from build123d import *

# Parameters (mm, degrees)
EXTRUDE_1_DEPTH      = 5
SKETCH_2_R           = 3.25
CUT_EXTRUDE_1_DEPTH  = 5
SKETCH_10_R          = 1.75
CUT_EXTRUDE_8_DEPTH  = 45
SKETCH_11_R          = 3.5
CUT_EXTRUDE_9_DEPTH  = 3
SKETCH_12_W          = 44
SKETCH_12_H          = 44
CUT_EXTRUDE_10_DEPTH = 5
SKETCH_13_W          = 44
SKETCH_13_H          = 44
EXTRUDE_2_DEPTH      = 16
EXTRUDE_3_DEPTH      = 4
FILLET_1_R           = 5
SKETCH_16_R          = 11.5
CUT_EXTRUDE_11_DEPTH = 3
SKETCH_17_R          = 3
CUT_EXTRUDE_12_DEPTH = 3
FILLET_2_R           = 5
SKETCH_20_R          = 3
CUT_EXTRUDE_14_DEPTH = 39
EXTRUDE_START        = 20
SKETCH_21_R          = 4.5
SKETCH_21_R_2        = 3
EXTRUDE_4_DEPTH      = 20
CHAMFER_1_SIZE       = 10
CHAMFER_1_SIZE2      = 17.320508076
SKETCH_22_R          = 10
CUT_EXTRUDE_15_DEPTH = 2
SKETCH_23_R          = 4.5
CUT_EXTRUDE_16_DEPTH = 5


with BuildPart() as part:
    # 草图1 → 凸台-拉伸1 (new body)
    with BuildSketch(Plane(origin=(0, 0, 0), x_dir=(1, 0, 0), z_dir=(0, 1, 0))):
        with BuildLine():
            Line((-40, 104.403065089), (-40, 230))
            ThreePointArc((-40, 230), (0, 270), (40, 230))
            Line((40, 230), (40, 104.403065089))
            ThreePointArc((40, 104.403065089), (42.277916175, 56.729935627), (49.090909091, 9.491187735))
            ThreePointArc((49.090909091, 9.491187735), (0, -50), (-49.090909091, 9.491187735))
            ThreePointArc((-49.090909091, 9.491187735), (-42.277916175, 56.729935627), (-40, 104.403065089))
        make_face()
    extrude(amount=EXTRUDE_1_DEPTH)

    # 草图2 → 切除-拉伸1 (cut)
    with BuildSketch(Plane(origin=(0, 5, 0), x_dir=(1, 0, 0), z_dir=(0, 1, 0))):
        with Locations(Location((28.284271247, 28.284271247, 0), (0, 0, 270))):
            Circle(SKETCH_2_R)
        with Locations(Location((28.284271247, -28.284271247, 0), (0, 0, 270))):
            Circle(SKETCH_2_R)
        with Locations(Location((-28.284271247, -28.284271247, 0), (0, 0, 270))):
            Circle(SKETCH_2_R)
        with Locations(Location((-28.284271247, 28.284271247, 0), (0, 0, 270))):
            Circle(SKETCH_2_R)
    extrude(amount=-CUT_EXTRUDE_1_DEPTH, mode=Mode.SUBTRACT)

    # 草图10 → 切除-拉伸8 (cut)
    with BuildSketch(Plane.XZ):
        with Locations(Location((46, 0, 0), (0, 0, 270))):
            Circle(SKETCH_10_R)
        with Locations(Location((36, -104.403065089, 0), (0, 0, 270))):
            Circle(SKETCH_10_R)
        with Locations(Location((36, -230, 0), (0, 0, 270))):
            Circle(SKETCH_10_R)
        with Locations(Location((-36, -230, 0), (0, 0, 270))):
            Circle(SKETCH_10_R)
        with Locations(Location((-36, -104.403065089, 0), (0, 0, 270))):
            Circle(SKETCH_10_R)
        with Locations(Location((-46, 0, 0), (0, 0, 270))):
            Circle(SKETCH_10_R)
    extrude(amount=-CUT_EXTRUDE_8_DEPTH, mode=Mode.SUBTRACT)

    # 草图11 → 切除-拉伸9 (cut)
    with BuildSketch(Plane(origin=(0, 5, 0), x_dir=(1, 0, 0), z_dir=(0, 1, 0))):
        with Locations(Location((-36, 230, 0), (0, 0, 270))):
            Circle(SKETCH_11_R)
        with Locations(Location((-36, 104.403065089, 0), (0, 0, 270))):
            Circle(SKETCH_11_R)
        with Locations(Location((-46, 0, 0), (0, 0, 270))):
            Circle(SKETCH_11_R)
        with Locations(Location((46, 0, 0), (0, 0, 90))):
            Circle(SKETCH_11_R)
        with Locations(Location((36, 104.403065089, 0), (0, 0, 90))):
            Circle(SKETCH_11_R)
        with Locations(Location((36, 230, 0), (0, 0, 90))):
            Circle(SKETCH_11_R)
    extrude(amount=-CUT_EXTRUDE_9_DEPTH, mode=Mode.SUBTRACT)

    # 草图12 → 切除-拉伸10 (cut)
    with BuildSketch(Plane(origin=(0, 5, 0), x_dir=(1, 0, 0), z_dir=(0, 1, 0))):
        with Locations((0, -4)):
            Rectangle(SKETCH_12_W, SKETCH_12_H)
    extrude(amount=-CUT_EXTRUDE_10_DEPTH, mode=Mode.SUBTRACT)

    # 草图13 → 凸台-拉伸2 (add)
    with BuildSketch(Plane.XZ):
        with BuildLine():
            Line((-21, 30), (21, 30))
            ThreePointArc((21, 30), (24.535533906, 28.535533906), (26, 25))
            Line((26, 25), (26, -17))
            ThreePointArc((26, -17), (24.535533906, -20.535533906), (21, -22))
            Line((21, -22), (-21, -22))
            ThreePointArc((-21, -22), (-24.535533906, -20.535533906), (-26, -17))
            Line((-26, -17), (-26, 25))
            ThreePointArc((-26, 25), (-24.535533906, 28.535533906), (-21, 30))
        make_face()
        with Locations((0, 4)):
            Rectangle(SKETCH_13_W, SKETCH_13_H, mode=Mode.SUBTRACT)
    extrude(amount=EXTRUDE_2_DEPTH)

    # 草图15 → 凸台-拉伸3 (add)
    with BuildSketch(Plane.XZ.offset(16)):
        with BuildLine():
            Line((26, -17), (26, 25))
            ThreePointArc((26, 25), (24.535533906, 28.535533906), (21, 30))
            Line((21, 30), (-21, 30))
            ThreePointArc((-21, 30), (-24.535533906, 28.535533906), (-26, 25))
            Line((-26, 25), (-26, -17))
            ThreePointArc((-26, -17), (-24.535533906, -20.535533906), (-21, -22))
            Line((-21, -22), (21, -22))
            ThreePointArc((21, -22), (24.535533906, -20.535533906), (26, -17))
        make_face()
    extrude(amount=EXTRUDE_3_DEPTH)

    # 圆角1
    fillet_1_edges = [part.edges().sort_by_distance(p)[0] for p in [
        (24.535533906, -20, 28.535533906),
        (0, -20, 30),
        (-24.535533906, -20, 28.535533906),
        (-26, -20, 4),
        (-24.535533906, -20, -20.535533906),
        (0, -20, -22),
        (24.535533906, -20, -20.535533906),
        (26, -20, 4),
    ]]
    fillet(fillet_1_edges, radius=FILLET_1_R)

    # 草图16 → 切除-拉伸11 (cut)
    with BuildSketch(Plane(origin=(0, -16, 0), x_dir=(1, 0, 0), z_dir=(0, 1, 0))):
        with Locations(Location((0, -4, 0), (0, 0, 270))):
            Circle(SKETCH_16_R)
    extrude(amount=-CUT_EXTRUDE_11_DEPTH, mode=Mode.SUBTRACT)

    # 草图17 → 切除-拉伸12 (cut)
    with BuildSketch(Plane(origin=(0, -19, 0), x_dir=(1, 0, 0), z_dir=(0, 1, 0))):
        with Locations(Location((0, -4, 0), (0, 0, 270))):
            Circle(SKETCH_17_R)
    extrude(amount=-CUT_EXTRUDE_12_DEPTH, mode=Mode.SUBTRACT)

    # 圆角2
    fillet_2_edges = [part.edges().sort_by_distance(p)[0] for p in [
        (22, -5.5, -18),
        (22, -5.5, 26),
        (-22, -5.5, 26),
        (-22, -5.5, -18),
    ]]
    fillet(fillet_2_edges, radius=FILLET_2_R)

    # 草图20 → 切除-拉伸14 (cut)
    with BuildSketch(Plane.XZ):
        with Locations(Location((0, -230, 0), (0, 0, 270))):
            Circle(SKETCH_20_R)
    extrude(amount=-CUT_EXTRUDE_14_DEPTH, mode=Mode.SUBTRACT)

    # 草图21 → 凸台-拉伸4 (add)
    with BuildSketch(Plane.XZ.offset(EXTRUDE_START)):
        with Locations(Location((0, -230, 0), (0, 0, 270))):
            Circle(SKETCH_21_R)
        with Locations(Location((0, -230, 0), (0, 0, 270))):
            Circle(SKETCH_21_R_2, mode=Mode.SUBTRACT)
    extrude(amount=-EXTRUDE_4_DEPTH)

    # 倒角1
    chamfer_1_edges = [part.edges().sort_by_distance(p)[0] for p in [
        (0, 0, -225.5),
    ]]
    chamfer_1_side = [part.faces().sort_by_distance(p)[0] for p in [
        (0, 0, -117.507600063),
    ]]
    chamfer(chamfer_1_edges, length=CHAMFER_1_SIZE, length2=CHAMFER_1_SIZE2, reference=chamfer_1_side[0])

    # 草图22 → 切除-拉伸15 (cut)
    with BuildSketch(Plane(origin=(0, 5, 0), x_dir=(1, 0, 0), z_dir=(0, 1, 0))):
        with Locations(Location((0, 230, 0), (0, 0, 270))):
            Circle(SKETCH_22_R)
    extrude(amount=-CUT_EXTRUDE_15_DEPTH, mode=Mode.SUBTRACT)

    # 草图23 → 切除-拉伸16 (cut)
    with BuildSketch(Plane(origin=(0, 5, 0), x_dir=(1, 0, 0), z_dir=(0, 1, 0))):
        with Locations(Location((0, 28.284271247, 0), (0, 0, 270))):
            Circle(SKETCH_23_R)
    extrude(amount=-CUT_EXTRUDE_16_DEPTH, mode=Mode.SUBTRACT)


solid = part.part
CAD build for the part. Positions are in the model's coordinates, mm. A direction names the side the tool comes from. Coordinates: 2 decimals unless noted, no trailing zeros. Order: outer loops, then holes, each group sorted by start corner. A loop starts at its lowest first (then second) coordinate and runs counter-clockwise, first axis right, second up. Notation, with made-up numbers: (11.5, -39.75) -> (29.5, -39.75) arc R17 cw to (29.5, -34.75) -> close; hole circle Ø4 at (66, 22). An arc over 180 degrees is marked (long way). Answer in a Markdown table with one row per item.
1) Band-saw the part on B-B (z = -208). List the corners of the cut face in (x, y).
Check values:
| item | result |
|---|---|
| outline | (-40, 0) -> (40, 0) -> (40, 5) -> (-40, 5) -> close |
2) Flat gauge pins, fed straight in: P1, Ø1.5, axis at x = -29, z = -196, coming from the -Y side; P2, Ø2, axis at x = -44.5, z = -0.5, coming from the +Y side; P3, Ø10.5, axis at y = -5, z = 9, coming from the -X side. Where does each tip first touch, or does it go through?
Check values:
| item | result |
|---|---|
| P1 | y = 0 |
| P2 | y = 2 |
| P3 | x = -49.45 |
3) Band-saw the part on A-A (y = -11.5). List the corners of the cut face in (x, z).
Check values:
| item | result |
|---|---|
| outline | (-26, -17) arc R5 ccw to (-21, -22) -> (21, -22) arc R5 ccw to (26, -17) -> (26, 25) arc R5 ccw to (21, 30) -> (-21, 30) arc R5 ccw to (-26, 25) -> close; circle Ø15.72 at (0, -230); hole (-22, -13) arc R5 ccw to (-17, -18) -> (17, -18) arc R5 ccw to (22, -13) -> (22, 21) arc R5 ccw to (17, 26) -> (-17, 26) arc R5 ccw to (-22, 21) -> close; hole circle Ø6 at (0, -230) |
4) Mould opens along Z. For faces 4 (the face through (0, -7, -22)), 5 (the face through (-0.88, 2.46, -269.99)), 6 (the face through (0, -20, 9)) say: pulls with the +Z half, pulls with the -Z half, needs draft (parallel to the pull), parting line crosses it, or undercut.
Check values:
| item | result |
|---|---|
| face 4 | undercut |
| face 5 | pulls with the -Z half |
| face 6 | needs draft |
5) Drill centre lines: line 1 (X direction, y = 3.3, z = -230); line 2 (Z direction, x = 4, y = -9.5); line 3 (Z direction, x = 36, y = 3). Where is each one in solid material? Low to high.
Check values:
| item | result |
|---|---|
| line 1 | -40 to -39.5, -32.5 to -10, 10 to 32.5, 39.5 to 40 |
| line 2 | -238.08 to -221.92, -22 to -18, 26 to 30 |
| line 3 | -247.44 to -233.5, -226.5 to -107.9, -100.9 to 34.7 |
6) Which spindle directions (+Z, -Z, +X, -X, +Y, -Y) get a long thin tool onto all of the face, cutting with end or side? Do faces 1 (the face through (0, -7, 30)), 2 (the face through (-42.342, 2.465, -56.065)), 3 (the face through (-32.53, 3.52, -230.46)). Say none if no direction does.
Check values:
| item | result |
|---|---|
| face 1 | +Z, +X, -X, -Y |
| face 2 | -Z, -X, +Y, -Y |
| face 3 | +Y |
7) Band-saw the part on C-C (z = -68.5). List the corners of the cut face in (x, y), and give its area (3 significant figures).
Check values:
| item | result |
|---|---|
| outline | (-41.29, 0) -> (41.29, 0) -> (41.29, 5) -> (-41.29, 5) -> close |
| area | 413 mm2 |
